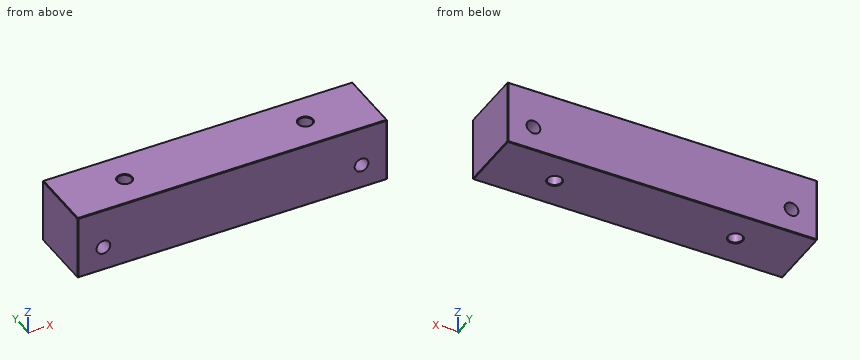
```python
from build123d import *

# Parameters (mm, degrees)
SKETCH1_W             = 60.96
SKETCH1_H             = 12.7
BOSS_EXTRUDE1_DEPTH   = 6.35
F_6_32_TAPPED_HOLE1_D = 2.7051
F_6_32_TAPPED_HOLE2_D = 2.7051
CHAMFER1_SIZE         = 0.127


with BuildPart() as part:
    # Sketch1 → Boss-Extrude1 (new body, symmetric)
    with BuildSketch(Plane(origin=(0, 0, 0), x_dir=(1, 0, 0), z_dir=(0, 1, 0))):
        Rectangle(SKETCH1_W, SKETCH1_H)
    extrude(amount=BOSS_EXTRUDE1_DEPTH, both=True)

    # #6-32 Tapped Hole1 (through all)
    with Locations(Plane(origin=(0, 6.35, 0), x_dir=(1, 0, 0), z_dir=(0, 1, 0))):
        with Locations((-25.4, 1.524), (25.4, 1.524)):
            Hole(F_6_32_TAPPED_HOLE1_D / 2)

    # #6-32 Tapped Hole2 (through all)
    with Locations(Plane.XY.offset(6.35)):
        with Locations((-17.78, 0), (17.78, 0)):
            Hole(F_6_32_TAPPED_HOLE2_D / 2)

    # Chamfer1
    chamfer1_edges = [part.edges().sort_by_distance(p)[0] for p in [
        (-30.48, 6.35, 0),
        (0, 6.35, 6.35),
        (19.13255, 0, 6.35),
        (19.13255, 0, -6.35),
        (-16.42745, 0, 6.35),
        (-16.42745, 0, -6.35),
        (30.48, 6.35, 0),
        (0, -6.35, 6.35),
        (-30.48, -6.35, 0),
        (0, -6.35, -6.35),
        (30.48, -6.35, 0),
        (0, 6.35, -6.35),
        (30.48, 0, 6.35),
        (-30.48, 0, 6.35),
        (-30.48, 0, -6.35),
        (30.48, 0, -6.35),
    ]]
    chamfer(chamfer1_edges, length=CHAMFER1_SIZE)


solid = part.part
```
Geometry: final body of the model. Coordinates: model frame, mm. Coordinates: 2 decimals unless noted, no trailing zeros. Order: outer loops, then holes, each group sorted by start corner. A loop starts at its lowest first (then second) coordinate and runs counter-clockwise, first axis right, second up. Notation, with made-up numbers: (-40, 75) -> (-22, 75) arc R23 cw to (-22, 98) -> close; hole circle Ø10 at (15, -16). An arc over 180 degrees is marked (long way). Write each question's results on one line, items separated by ' | '. Start each with the question number.
1) Cut plane B-B, the plane y = 0. Output: boundary loops of the cut face in (x, z), and give its area (3 significant figures).
2) Cut plane A-A, the plane z = -1. Output: boundary loops of the cut face in (x, y), and give its area (3 significant figures).
3) Cut plane C-C, the plane x = 25.4. Output: boundary loops of the cut face in (y, z).
4) Cut plane D-D, the plane x = -17.78. Output: boundary loops of the cut face in (y, z).
5) Material intervals for line 1 along Z through (x, y) = (-25.4, -2.5); line 2 along X through (y, z) = (0.5, 4.5), sorted ascending.
Checks:
1) outline: (-30.48, -6.22) -> (-30.35, -6.35) -> (-19.26, -6.35) -> (-19.13, -6.22) -> (-19.13, 6.22) -> (-19.26, 6.35) -> (-30.35, 6.35) -> (-30.48, 6.22) -> close; (-16.43, -6.22) -> (-16.3, -6.35) -> (16.3, -6.35) -> (16.43, -6.22) -> (16.43, 6.22) -> (16.3, 6.35) -> (-16.3, 6.35) -> (-16.43, 6.22) -> close; (19.13, -6.22) -> (19.26, -6.35) -> (30.35, -6.35) -> (30.48, -6.22) -> (30.48, 6.22) -> (30.35, 6.35) -> (19.26, 6.35) -> (19.13, 6.22) -> close; hole circle Ø2.71 at (-25.4, -1.52); hole circle Ø2.71 at (25.4, -1.52) | area: 694 mm^2
2) outline: (-30.48, -6.22) -> (-30.35, -6.35) -> (-26.65, -6.35) -> (-26.65, 6.35) -> (-30.35, 6.35) -> (-30.48, 6.22) -> close; (-24.15, -6.35) -> (24.15, -6.35) -> (24.15, 6.35) -> (-24.15, 6.35) -> close; (26.65, -6.35) -> (30.35, -6.35) -> (30.48, -6.22) -> (30.48, 6.22) -> (30.35, 6.35) -> (26.65, 6.35) -> close; hole circle Ø2.71 at (-17.78, 0); hole circle Ø2.71 at (17.78, 0) | area: 699 mm^2
3) outline: (-6.35, -6.22) -> (-6.22, -6.35) -> (6.22, -6.35) -> (6.35, -6.22) -> (6.35, -2.88) -> (-6.35, -2.88) -> close; (-6.35, -0.17) -> (6.35, -0.17) -> (6.35, 6.22) -> (6.22, 6.35) -> (-6.22, 6.35) -> (-6.35, 6.22) -> close
4) outline: (-6.35, -6.22) -> (-6.22, -6.35) -> (-1.48, -6.35) -> (-1.35, -6.22) -> (-1.35, 6.22) -> (-1.48, 6.35) -> (-6.22, 6.35) -> (-6.35, 6.22) -> close; (1.35, -6.22) -> (1.48, -6.35) -> (6.22, -6.35) -> (6.35, -6.22) -> (6.35, 6.22) -> (6.22, 6.35) -> (1.48, 6.35) -> (1.35, 6.22) -> close
5) line 1: -6.35 to -2.88, -0.17 to 6.35 | line 2: -30.48 to -19.04, -16.52 to 16.52, 19.04 to 30.48
